from build123d import *

# Parameters (mm, degrees)
BOSS_EXTRUDE1_DEPTH = 15
SKETCH2_R           = 3
CUT_EXTRUDE1_DEPTH  = 17
SKETCH3_R           = 3
CUT_EXTRUDE2_DEPTH  = 17


with BuildPart() as part:
    # Sketch1 → Boss-Extrude1 (new body)
    with BuildSketch(Plane.XY):
        Polygon((-30.175322727, 12.351876728), (-30.175322727, -7.648123272), (-15.175322727, -7.648123272), (-15.175322727, 12.351876728), (-17.675322727, 12.351876728), (-17.675322727, -5.148123272), (-27.675322727, -5.148123272), (-27.675322727, 12.351876728), align=None)
    extrude(amount=BOSS_EXTRUDE1_DEPTH)

    # Sketch2 → Cut-Extrude1 (cut)
    with BuildSketch(Plane(origin=(-15.175322727, 0, 0), x_dir=(0, 0, -1), z_dir=(1, 0, 0))):
        with Locations((-7.5, 7.104053692)):
            Circle(SKETCH2_R)
    extrude(amount=-CUT_EXTRUDE1_DEPTH, mode=Mode.SUBTRACT)

    # Sketch3 → Cut-Extrude2 (cut)
    with BuildSketch(Plane(origin=(0, -7.648123272, 0), x_dir=(-1, 0, 0), z_dir=(0, -1, 0))):
        with Locations(Location((22.675322727, -7.5, 0), (0, 0, 90))):
            Circle(SKETCH3_R)
    extrude(amount=-CUT_EXTRUDE2_DEPTH, mode=Mode.SUBTRACT)


solid = part.part
Read the model definition and answer for the solid it produces. Units are mm, in the model's axes. A direction names the side the tool comes from. Give positions to 0.01 mm unless a question says otherwise; leave off trailing zeros. Write each loop counter-clockwise with the first axis right and the second up, starting at its lowest first coordinate (ties: lowest second). Pieces come first, ordered by that corner, then holes. Notation, with made-up numbers: (67.5, 38.5) - (98.5, 38.5) arc R11 cw to (98.5, 43.5) - close; hole circle Ø3 at (50.5, 83). An arc over 180 degrees is marked (long way). Answer in a Markdown table with one row per item. Add a question column.
Item 1: Find the intervals of material crossed by L1, parallel to X at y = -3.25, z = 9.5; L2, parallel to Y at x = -29, z = 7.5; L3, parallel to Y at x = -28.5, z = 5.5, in increasing order.
Item 2: Section C-C, the plane z = 12 is taken. Write down the section's boundary in (x, y), and give its area (3 significant figures).
Item 3: Section D-D, the plane x = -18.25 is taken. Write down the section's boundary in (y, z).
Item 4: Section B-B, the plane y = -0.75 is taken. Write down the section's boundary in (x, z), and give its area (3 significant figures).
Item 5: Section A-A, the plane z = 7.5 is taken. Write down the section's boundary in (x, y), and give its area (3 significant figures).
Item 6: A flat-ended cylindrical pin translates along its axis: P1, Ø5.5, axis at y = 7.1, z = 7.5, coming from the +X side. Find the tip coordinate at first contact, or state that the pin passes through.
Item 7: Determine the mould class of faces 3 (the face through (-17.675, 3.7, 7.4)), 4 (the face through (-15.175, 2, 7)), 5 (the face through (-16, 12.352, 7)) for opening direction X: pulls with the +X half, pulls with the -X half, needs draft (parallel to the pull), parting line crosses it, or undercut.
Item 8: A tool of negligible diameter and unlimited length cuts with its end or side. For faces 1 (the face through (-27.675, 3, 7)), 2 (the face through (-29, 12.352, 7)), from which of +Z, -Z, +X, -X, +Y, -Y can it reach the whole face along a straight path? Write none if from no direction.
Recorded:
| question | item | result |
|---|---|---|
| 1 | L1 | x = -30.18 to -27.68, -17.68 to -15.18 |
| 1 | L2 | y = -7.65 to 4.1, 10.1 to 12.35 |
| 1 | L3 | y = -7.65 to 4.87, 9.34 to 12.35 |
| 2 | outline | (-30.18, -7.65) - (-15.18, -7.65) - (-15.18, 12.35) - (-17.68, 12.35) - (-17.68, -5.15) - (-27.68, -5.15) - (-27.68, 12.35) - (-30.18, 12.35) - close |
| 2 | area | 125 mm2 |
| 3 | outline | (-7.65, 0) - (-5.15, 0) - (-5.15, 15) - (-7.65, 15) - close |
| 4 | outline | (-30.18, 0) - (-27.68, 0) - (-27.68, 15) - (-30.18, 15) - close; (-17.68, 0) - (-15.18, 0) - (-15.18, 15) - (-17.68, 15) - close |
| 4 | area | 75.0 mm2 |
| 5 | outline | (-30.18, -7.65) - (-25.68, -7.65) - (-25.68, -5.15) - (-27.68, -5.15) - (-27.68, 4.1) - (-30.18, 4.1) - close; (-30.18, 10.1) - (-27.68, 10.1) - (-27.68, 12.35) - (-30.18, 12.35) - close; (-19.68, -7.65) - (-15.18, -7.65) - (-15.18, 4.1) - (-17.68, 4.1) - (-17.68, -5.15) - (-19.68, -5.15) - close; (-17.68, 10.1) - (-15.18, 10.1) - (-15.18, 12.35) - (-17.68, 12.35) - close |
| 5 | area | 80.0 mm2 |
| 6 | P1 | passes through |
| 7 | face 3 | undercut |
| 7 | face 4 | pulls with the +X half |
| 7 | face 5 | needs draft |
| 8 | face 1 | +Z, -Z, +Y |
| 8 | face 2 | +Z, -Z, +X, -X, +Y |
